Check sheet for the drawn part. Datum: minimum x, y, z corner. Units: mm. Coordinates: 2 decimals unless noted, no trailing zeros. Write each loop counter-clockwise with the first axis right and the second up, starting at its lowest first coordinate (ties: lowest second). Pieces come first, ordered by that corner, then holes. Notation, with made-up numbers: (86.5, -30) -> (93.5, -30) arc R29 cw to (93.5, -6) -> close; hole circle Ø4 at (34.25, 85). An arc over 180 degrees is marked (long way). Answer in a Markdown table with one row per item. Add a question column.
1. Cross-section at B-B on x = 120. Record the cut outline in (y, z).
2. Cross-section at C-C on y = 10. Give the number of separate pieces and of enclosed holes in the cut face, and give its area (3 significant figures).
3. Scan lines: L1, parallel to Z at x = 323, y = 15; L2, parallel to X at y = 15, z = 51.5; L3, parallel to Y at x = 50, z = 4. Record each from-to range of solid material in increasing order. Write a range as from..to.
4. Cross-section at A-A on z = 271. Record the cut outline in (x, y).
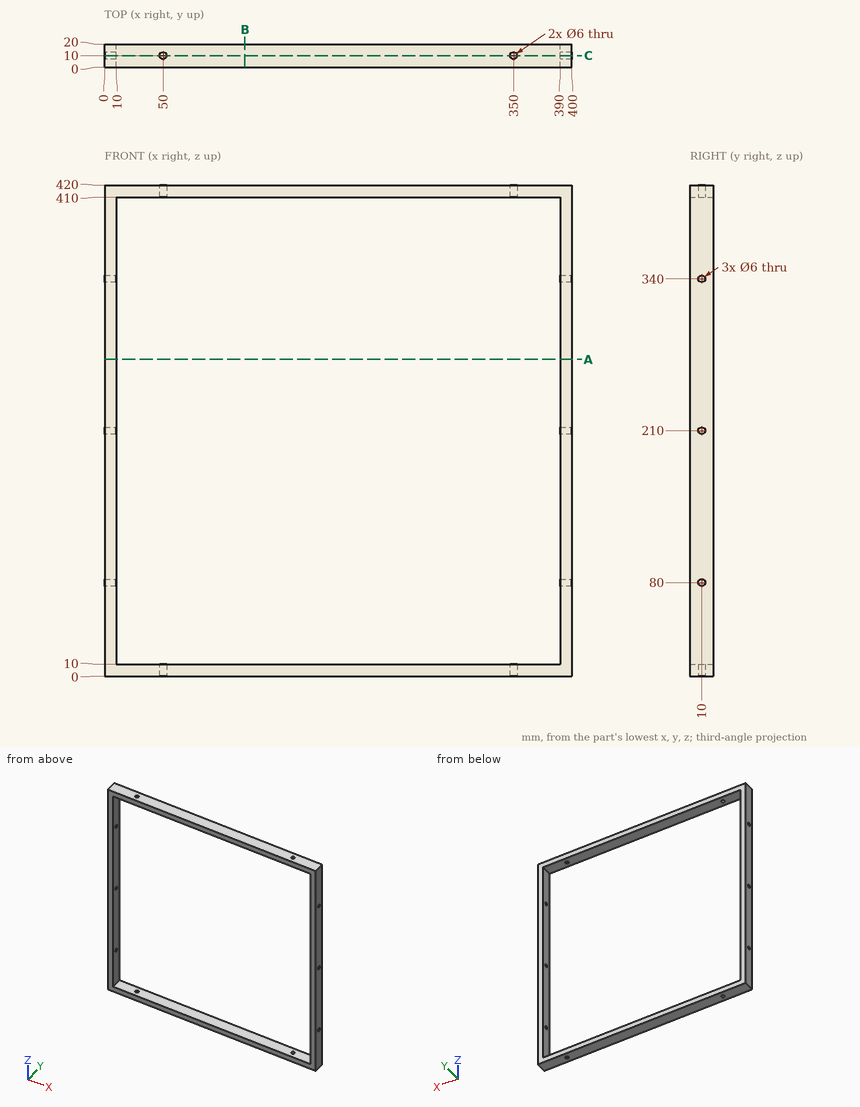
Results found:
| question | item | result |
|---|---|---|
| 1 | outline | (0, 0) -> (20, 0) -> (20, 10) -> (0, 10) -> close; (0, 410) -> (20, 410) -> (20, 420) -> (0, 420) -> close |
| 2 | separate pieces | 10 |
| 2 | enclosed holes | 0 |
| 2 | area | 15,400 mm^2 |
| 3 | L1 | z = 0..10, 410..420 |
| 3 | L2 | x = 0..10, 390..400 |
| 3 | L3 | y = 0..7, 13..20 |
| 4 | outline | (0, 0) -> (10, 0) -> (10, 20) -> (0, 20) -> close; (390, 0) -> (400, 0) -> (400, 20) -> (390, 20) -> close |
